The figure shows three views and two pictorial views of one solid part (mm, origin at its lowest corner). Answer the questions. A direction names the side the tool comes from. Give positions to 0.01 mm unless a question says otherwise; leave off trailing zeros. Order: outer loops, then holes, each group sorted by start corner. A loop starts at its lowest first (then second) coordinate and runs counter-clockwise, first axis right, second up. Notation, with made-up numbers: (4, 79) - (26, 79) arc R12 cw to (26, 97) - close; hole circle Ø5 at (19.5, 61). An arc over 180 degrees is marked (long way). Answer as a JSON object with one key per item and string values. Group by question number.
Q1. A cutting plane is placed at B-B, the plane z = 16.5. Give the vertices of the cut face in (x, y).
Q2. Consider line 1 (Y direction, x = 20, z = 13.5); line 2 (X direction, y = 52, z = 8.5); line 3 (Y direction, x = 36, z = 11.75). Determine where each line is inside the solid, lowest interval first.
Q3. A cutting plane is placed at A-A, the plane x = 30. Give the vertices of the cut face in (y, z).
Q4. For the marked faces 1 and 2, determine the directions among +Z, -Z, +X, -X, +Y, -Y from which every point of the face is accessible in a straight line to the end or side of a thin tool.
Q5. A cutting plane is placed at C-C, the plane y = 53.5. Give the vertices of the cut face in (x, z), and give its area (3 significant figures).
Q6. Given pin 1 (2.5 mm diameter, centred on x = 12.7, z = 9.525, fed in from +Y); pin 2 (1.6 mm diameter, centred on x = 6.35, z = 9.525, fed in from -Y) (1 decimal); pin 3 (5 mm diameter, centred on x = 17.5, z = 6, fed in from +Y), each flat-ended and moving along its own axis, determine where each tip first touches the part or whether it passes through.
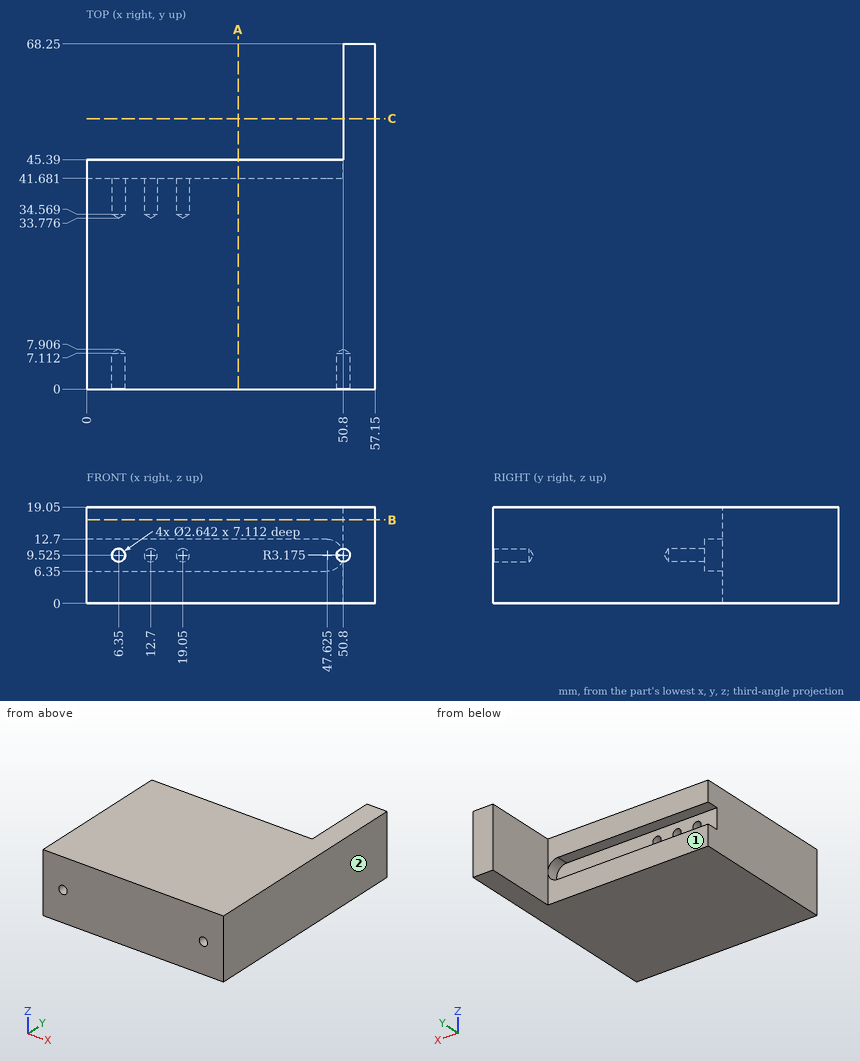
Reply:
{
 "1": {"outline": "(0, 0) - (57.15, 0) - (57.15, 68.25) - (50.8, 68.25) - (50.8, 45.39) - (0, 45.39) - close"},
 "2": {"line 1": "y = 0 to 45.39", "line 2": "x = 50.8 to 57.15", "line 3": "y = 0 to 41.68"},
 "3": {"outline": "(0, 0) - (45.39, 0) - (45.39, 6.35) - (41.68, 6.35) - (41.68, 12.7) - (45.39, 12.7) - (45.39, 19.05) - (0, 19.05) - close"},
 "4": {"face 1": "+Z, -Z, -X, +Y", "face 2": "+Z, -Z, +X, +Y, -Y"},
 "5": {"outline": "(50.8, 0) - (57.15, 0) - (57.15, 19.05) - (50.8, 19.05) - close", "area": "121 mm^2"},
 "6": {"pin 1": "stops at y = 34.53", "pin 2": "stops at y = 7.4", "pin 3": "stops at y = 45.39"}
}
